Design review of the part built by this model. Coordinates are the model's own, in mm. Coordinates: 2 decimals unless noted, no trailing zeros. Write each loop counter-clockwise with the first axis right and the second up, starting at its lowest first coordinate (ties: lowest second). Pieces come first, ordered by that corner, then holes. Notation, with made-up numbers: M -19,77 L 18,77 A21 cw 18,99 Z; hole C -0.75,44 d11. An arc over 180 degrees is marked long. Return JSON: item names as keys, results as strings. Group by question number.
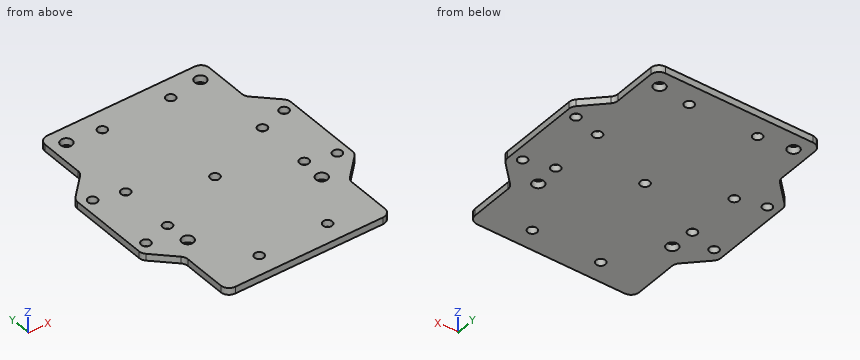
```python
from build123d import *

# Parameters (mm, degrees)
SKETCH1_W                  = 60
SKETCH1_H                  = 90
BOSS_EXTRUDE1_DEPTH        = 1.25
FILLET1_R                  = 3
F_4_2_4_2_DIAMETER_HOLE1_D = 4.2
M3_CLEARANCE_HOLE1_D       = 3.4
M3_CLEARANCE_HOLE2_D       = 3.4
M3_CLEARANCE_HOLE3_D       = 3.4


with BuildPart() as part:
    # Sketch1 → Boss-Extrude1 (new, symmetric)
    with BuildSketch(Plane.XY):
        Polygon((-30, 25), (-30, -25), (-30, -45), (30, -45), (30, -25), (30, 25), (30, 45), (-30, 45), align=None)
        Rectangle(SKETCH1_W, SKETCH1_H)
        Polygon((-39, 16), (-39, -16), (-30, -25), (-30, 25), align=None)
        Polygon((30, 25), (30, -25), (39, -16), (39, 16), align=None)
    extrude(amount=BOSS_EXTRUDE1_DEPTH, both=True)

    # Fillet1
    fillet1_edges = [part.edges().sort_by_distance(p)[0] for p in [
        (30, 25, 0),
        (39, 16, 0),
        (39, -16, 0),
        (30, -25, 0),
        (30, -45, 0),
        (-30, -45, 0),
        (-30, -25, 0),
        (-39, -16, 0),
        (-39, 16, 0),
        (-30, 25, 0),
        (-30, 45, 0),
        (30, 45, 0),
    ]]
    fillet(fillet1_edges, radius=FILLET1_R)

    # Ø4.2 (4.2) Diameter Hole1 (through all)
    with Locations(Plane(origin=(0, 0, -1.25), x_dir=(-1, 0, 0), z_dir=(0, 0, -1))):
        with Locations((-24.5, -19), (24.5, -19), (24.5, 39), (-24.5, 39)):
            Hole(F_4_2_4_2_DIAMETER_HOLE1_D / 2)

    # M3 Clearance Hole1 (through all)
    with Locations(Plane(origin=(0, 0, -1.25), x_dir=(-1, 0, 0), z_dir=(0, 0, -1))):
        with Locations((-35, 12.75), (-35, -12.75), (35, -12.75), (35, 12.75)):
            Hole(M3_CLEARANCE_HOLE1_D / 2)

    # M3 Clearance Hole2 (through all)
    with Locations(Plane.XY.offset(1.25)):
        with Locations((-12.5, -37.5), (12.5, -37.5), (-12.5, 37.5), (12.5, 37.5), (-25, 10), (-25, -10), (25, -10), (25, 10)):
            Hole(M3_CLEARANCE_HOLE2_D / 2)

    # M3 Clearance Hole3 (through all)
    with Locations(Plane.XY.offset(1.25)):
        with Locations((0, 0)):
            Hole(M3_CLEARANCE_HOLE3_D / 2)


solid = part.part
```
Item 1: Add section A-A (x = -35). Write out the cut boundary in (y, z), plus the area to 3 significant figures.
Item 2: Add section D-D (x = 0). Write out the cut boundary in (y, z), plus the area to 4 significant figures.
Item 3: For line 1 (Y direction, x = 12.5, z = -0.1); line 2 (Y direction, x = 35.5, z = 1); line 3 (Y direction, x = 26, z = -0.8), list the stretches that pass through material, from the lowest coordinate up.
Item 4: For pin 1 (2.5 mm diameter, centred on x = -12.5, y = -37.5, fed in from -Z); pin 2 (1.2 mm diameter, centred on y = -31.5, z = -0.5, fed in from +X); pin 3 (0.8 mm diameter, centred on y = 33.5, z = 0.5, fed in from -X), all flat-tipped, find the tip position at first contact; note any pin that passes through.
Item 5: Add section C-C (y = 0). Write out the cut boundary in (x, z), plus the area to 4 significant figures.
Item 6: Add section B-B (y = -37.5). Write out the cut boundary in (x, z), plus the area to 3 significant figures.
Geometry check:
{
 "1": {"outline": "M -20,-1.25 L -14.45,-1.25 L -14.45,1.25 L -20,1.25 Z; M -11.05,-1.25 L 11.05,-1.25 L 11.05,1.25 L -11.05,1.25 Z; M 14.45,-1.25 L 20,-1.25 L 20,1.25 L 14.45,1.25 Z", "area": "83.0 mm^2"},
 "2": {"outline": "M -45,-1.25 L -1.7,-1.25 L -1.7,1.25 L -45,1.25 Z; M 1.7,-1.25 L 45,-1.25 L 45,1.25 L 1.7,1.25 Z", "area": "216.5 mm^2"},
 "3": {"line 1": "-45 to -39.2, -35.8 to 35.8, 39.2 to 45", "line 2": "-19.5 to -14.37, -11.13 to 11.13, 14.37 to 19.5", "line 3": "-45 to -20.47, -17.53 to -11.37, -8.63 to 8.63, 11.37 to 37.53, 40.47 to 45"},
 "4": {"pin 1": "through", "pin 2": "x = 30", "pin 3": "x = -30"},
 "5": {"outline": "M -39,-1.25 L -1.7,-1.25 L -1.7,1.25 L -39,1.25 Z; M 1.7,-1.25 L 39,-1.25 L 39,1.25 L 1.7,1.25 Z", "area": "186.5 mm^2"},
 "6": {"outline": "M -30,-1.25 L -14.2,-1.25 L -14.2,1.25 L -30,1.25 Z; M -10.8,-1.25 L 10.8,-1.25 L 10.8,1.25 L -10.8,1.25 Z; M 14.2,-1.25 L 30,-1.25 L 30,1.25 L 14.2,1.25 Z", "area": "133 mm^2"}
}
